For this review, take the finished solid that the model builds, in its own axes (mm). Face numbers are marked on the shaded views. Give positions to 0.01 mm unless a question says otherwise; leave off trailing zeros. Write each loop counter-clockwise with the first axis right and the second up, starting at its lowest first coordinate (ties: lowest second). Pieces come first, ordered by that corner, then holes. Notation, with made-up numbers: (-15.5, 89.25) -> (33.5, 89.25) arc R9 ccw to (33.5, 98.25) -> close; hole circle Ø6 at (24, 39). An arc over 180 degrees is marked (long way). Answer as CSV lines item,"result".
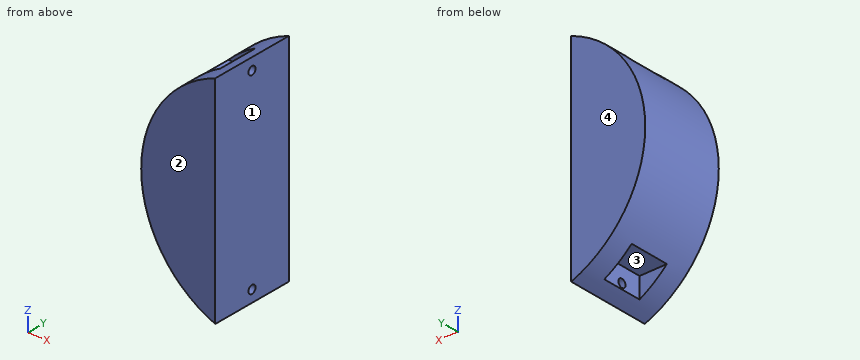
Autodesk Inventor part; units mm, degrees
ref_plane "РабПлоскость1" through (-42.5, 0, 0) normal (1, 0, 0) x (0, 1, 0)
ref_plane "YZ Plane" through (0, 0, 0) normal (1, 0, 0) x (0, 1, 0)
ref_plane "XZ Plane" through (0, 0, 0) normal (0, 1, 0) x (-1, 0, 0)
sketch "Эскиз1" plane through (0, 0, 0) normal (0, 1, 0) x (-1, 0, 0)
  circle A0 centre (0, 0) radius 3.9
  line L0 (-35, -37.5) -> (-35, 37.5)
  line L1 (-35, -37.5) -> (15, -37.5)
  line L2 (15, -37.5) -> (15, -39.7649)
  arc A1 (15, -39.7649) -> (15, 39.7649) centre (0, 0) ccw
  line L3 (15, 39.7649) -> (15, 37.5)
  line L4 (-35, 37.5) -> (15, 37.5)
  line L5 (15, 39.7649) -> (15, -39.7649)
  point P0 (-39, 0)
extrude "Выдавливание1" add sketch "Эскиз1" along normal blind 31.32 contours L5 L3 A1 L2
ref_plane "РабПлоскость1" through (-42.5, 0, 0) normal (1, 0, 0) x (0, 1, 0)
sketch "Эскиз2" plane through (-42.5, 0, 0) normal (1, 0, 0) x (0, 1, 0)
  line L0 (31.32, -39.7649) -> (31.32, 39.7649)
  line L1 (31.32, -39.7649) -> (15.66, -39.7649)
  line L2 (0, -39.7649) -> (31.32, -39.7649)
  line L3 (15.66, -39.7649) -> (15.66, -34.7649)
  line L4 (8.16, -39.7649) -> (23.16, -39.7649)
  line L5 (23.16, -39.7649) -> (23.16, -29.7649)
  line L6 (23.16, -29.7649) -> (8.16, -29.7649)
  line L7 (8.16, -29.7649) -> (8.16, -39.7649)
  line L8 (8.16, -39.7649) -> (23.16, -29.7649) construction
  line L9 (23.16, -39.7649) -> (8.16, -29.7649) construction
  line L10 (31.32, 0) -> (24.2001, 0)
  line L11 (31.32, 39.7649) -> (15.66, 39.7649)
  line L12 (0, 39.7649) -> (31.32, 39.7649)
  line L13 (15.66, 39.7649) -> (15.66, 34.7649)
  line L14 (8.16, 39.7649) -> (23.16, 39.7649)
  line L15 (23.16, 39.7649) -> (23.16, 29.7649)
  line L16 (23.16, 29.7649) -> (8.16, 29.7649)
  line L17 (8.16, 29.7649) -> (8.16, 39.7649)
  line L18 (8.16, 39.7649) -> (23.16, 29.7649) construction
  line L19 (23.16, 39.7649) -> (8.16, 29.7649) construction
  point P0 (0, 0)
  dimension "d2" = 15.66
  dimension "d3" = 5
  dimension "d4" = 15
  dimension "d5" = 10
extrude "Выдавливание2" cut sketch "Эскиз2" along normal blind 22.32
sketch "Эскиз3" plane through (-42.5, 0, 0) normal (1, 0, 0) x (0, 1, 0)
  line L0 (8.16, -37.4034) -> (23.16, -37.4034)
  line L1 (15.66, -37.4034) -> (15.66, -35.4034)
  circle A0 centre (15.66, -35.4034) radius 1.5
  line L2 (23.16, 37.4034) -> (8.16, 37.4034)
  line L3 (15.66, 37.4034) -> (15.66, 35.4034)
  circle A1 centre (15.66, 35.4034) radius 1.5
  point P0 (0, 0)
  dimension "d8" = 2
  dimension "d9" = 3
  dimension "d10" = 2
  dimension "d11" = 3
extrude "Выдавливание3" cut sketch "Эскиз3" along normal through all
properties part number "joint3_cap"
Q1. Add section C-C (x = -24). Write out the cut boundary in (y, z), plus the area to 3 significant figures.
Answer block:
outline,"(0, -35.07) -> (8.16, -35.07) -> (8.16, -29.76) -> (23.16, -29.76) -> (23.16, -35.07) -> (31.32, -35.07) -> (31.32, 35.07) -> (23.16, 35.07) -> (23.16, 29.76) -> (8.16, 29.76) -> (8.16, 35.07) -> (0, 35.07) -> close"
area,"2,040 mm2"
Q2. To check wall thickness, follow probe 1 along Z at (x, y) = (-16.9, 15.66); probe 2 along Z at (x, y) = (-17.3, 15.66); probe 3 along X at (y, z) = (13, -33.5). State the ranges of each line that lie inside material, in increasing order. Write a range as [from, to].
Answer block:
probe 1,"z = [-39, -36.9], [-33.9, 33.9], [36.9, 39]"
probe 2,"z = [-38.82, -36.9], [-33.9, 33.9], [36.9, 38.82]"
probe 3,"x = [-20.18, -15]"
Q3. Add section D-D (z = 15). Write out the cut boundary in (x, y), plus the area to 3 significant figures.
Answer block:
outline,"(-39.76, 0) -> (-15, 0) -> (-15, 31.32) -> (-39.76, 31.32) -> close"
area,"776 mm2"
Q4. Add section A-A (y = 10.5). Write out the cut boundary in (x, z).
Answer block:
outline,"(-30.34, -29.76) -> (-20.18, -29.76) -> (-20.18, -37.4) arc R42.5 ccw to (-15, -39.76) -> (-15, 39.76) arc R42.5 ccw to (-20.18, 37.4) -> (-20.18, 29.76) -> (-30.34, 29.76) arc R42.5 ccw to start"
Q5. Add section B-B (y = 15.66). Write out the cut boundary in (x, z).
Answer block:
outline,"(-30.34, -29.76) -> (-20.18, -29.76) -> (-20.18, -33.9) -> (-15, -33.9) -> (-15, 33.9) -> (-20.18, 33.9) -> (-20.18, 29.76) -> (-30.34, 29.76) arc R42.5 ccw to start; (-20.18, -37.4) arc R42.5 ccw to (-15, -39.76) -> (-15, -36.9) -> (-20.18, -36.9) -> close; (-20.18, 36.9) -> (-15, 36.9) -> (-15, 39.76) arc R42.5 ccw to (-20.18, 37.4) -> close"
Q6. Draft analysis for pull direction Y (two halves, no side actions). For the marked faces 1, 2, 3 and 4, state which applies: released by +Y, released by -Y, zero draft, split by the parting line, or undercut.
Answer block:
face 1,"zero draft"
face 2,"released by -Y"
face 3,"undercut"
face 4,"released by +Y"
Q7. Clearance check with flat-ended pins moving along their axes: pin 1 (1 mm diameter, centred on x = -19.5, y = 12, fed in from +Z); pin 2 (8 mm diameter, centred on x = -23, y = 16.5, fed in from -Z); pin 3 (2.5 mm diameter, centred on y = 15.66, z = -35.4, fed in from +X); pin 4 (3 mm diameter, centred on x = -32, y = 17, fed in from +Z). State where each tip first meets the part, or that it passes through.
Answer block:
pin 1,"stops at z = 38.02"
pin 2,"stops at z = -38.02"
pin 3,"passes through"
pin 4,"stops at z = 29.6"
